Source: CAD feature listing. Evaluate the final solid. Frame: model axes, mm. A direction names the side the tool comes from. Give positions to 0.01 mm unless a question says otherwise; leave off trailing zeros. Write each loop counter-clockwise with the first axis right and the second up, starting at its lowest first coordinate (ties: lowest second). Pieces come first, ordered by that corner, then holes. Notation, with made-up numbers: (-13, 54) -> (21, 54) arc R28 cw to (21, 76) -> close; hole circle Ø9 at (-6.75, 55.5). An arc over 180 degrees is marked (long way). Use one line per item in the form item = value. Start each with the question number.
(1) Set-up query: faces 1 (the face through (-5, -2, 4)), 2 (the face through (-1.873, 3.367, 2.986)), 3 (the face through (-4.825, -7.192, 3.598)). Return all of +Z, -Z, +X, -X, +Y, -Y with unobstructed straight access to the full face (end or side cutting, diameter ignored); none if empty.
(2) Cut plane A-A, the plane z = 3.25. Count the separate pieces of the cut face and the enclosed holes in it, and give its area (3 significant figures).
(3) Material intervals for line 1 along Y through (x, z) = (-3, 1.75); line 2 along Z through (x, y) = (-3.5, 2.5); line 3 along Z through (x, y) = (-5.25, 8), sorted ascending. Write a range as from..to.
(4) Draft query along Z for faces 4 (the face through (-5, -2, 2)), 5 (the face through (-5.492, 5.648, 3.395)), 6 (the face through (-1.374, -10.002, 1.118)), 7 (the face through (-3.202, -7.94, 4.791)). Return one class per face: pulls with the +Z half, pulls with the -Z half, needs draft (parallel to the pull), parting line crosses it, or undercut.
(5) First-contact query: P1, Ø3, axis at x = -5.5, y = -9, coming from the -Z side; P2, Ø1.5, axis at y = -6, z = 5, coming from the +X side; P3, Ø1.6, axis at x = -3, y = 1, coming from the +Z side; P4, Ø4, axis at x = -3.5, y = -0.5, coming from the -Z side. Flat tips, straight axial feed; report the tip coordinate or a pass-through.
(6) Cut plane C-C, the plane x = -8.75. Output: boundary loops of the cut face in (y, z), and give its area (3 significant figures).
(7) Cut plane D-D, the plane y = -6. Output: boundary loops of the cut face in (x, z), and give its area (3 significant figures).
from build123d import *

# Parameters (mm, degrees)
BOSS_EXTRUDE2_DEPTH = 7
BOSS_EXTRUDE3_START = -2
BOSS_EXTRUDE3_DEPTH = 2
CUT_EXTRUDE1_REACH  = 20.032
SKETCH4_R           = 2.165
SKETCH6_R           = 3
CUT_EXTRUDE2_DEPTH  = 2.25


with BuildPart() as part:
    # Sketch2 → Boss-Extrude2 (new body)
    with BuildSketch(Plane.XY):
        with BuildLine():
            Line((-1.537034244, -5.640729849), (-1.207226003, -14.487186411))
            Line((-1.207226003, -14.487186411), (-7.804400539, -6.252306152))
            ThreePointArc((-7.804400539, -6.252306152), (-10, 0), (-7.804400539, 6.252306152))
            Line((-7.804400539, 6.252306152), (-2.239666493, 13.198449277))
            Line((-2.239666493, 13.198449277), (-1.909690796, 4.352324093))
            ThreePointArc((-1.909690796, 4.352324093), (-6.719838781, -0.830529263), (-1.537034244, -5.640729849))
        make_face()
    extrude(amount=BOSS_EXTRUDE2_DEPTH)

    # Sketch3 → Boss-Extrude3 (add)
    with BuildSketch(Plane.XY.offset(4).offset(BOSS_EXTRUDE3_START)):
        with BuildLine():
            Line((-1.909780577, 4.352320743), (-1.835249267, 2.353709953))
            ThreePointArc((-1.835249267, 2.353709953), (-4.721227993, -0.755997952), (-1.611655337, -3.642122406))
            Line((-1.611655337, -3.642122406), (-1.537124027, -5.640733196))
            ThreePointArc((-1.537124027, -5.640733196), (-6.719838781, -0.830529263), (-1.909780577, 4.352320743))
        make_face()
    extrude(amount=BOSS_EXTRUDE3_DEPTH)

    # Sketch4 → Cut-Extrude1 (cut, up to next)
    with BuildSketch(Plane(origin=(-1.744913711, -0.065088285, 0), x_dir=(0, 0, -1), z_dir=(0.9993050159682331, 0.03727579725142651, 0)), mode=Mode.PRIVATE) as cut_extrude1_sk1:
        with Locations(Location((-3.5, 8.846623232, 0), (0, 0, 90))):
            Circle(SKETCH4_R)
    cut_extrude1_tool1 = extrude(cut_extrude1_sk1.sketch, amount=-CUT_EXTRUDE1_REACH, mode=Mode.PRIVATE) & part.part
    # Sketch4 → Cut-Extrude1 (cut, up to next)
    with BuildSketch(Plane(origin=(-1.744913711, -0.065088285, 0), x_dir=(0, 0, -1), z_dir=(0.9993050159682331, 0.03727579725142651, 0)), mode=Mode.PRIVATE) as cut_extrude1_sk2:
        with Locations(Location((-3.5, -10.005816596, 0), (0, 0, 90))):
            Circle(SKETCH4_R)
    cut_extrude1_tool2 = extrude(cut_extrude1_sk2.sketch, amount=-CUT_EXTRUDE1_REACH, mode=Mode.PRIVATE) & part.part
    add(cut_extrude1_tool1.solids().sort_by_distance((-2.074679, 8.775387, 3.5))[0], mode=Mode.SUBTRACT)
    add(cut_extrude1_tool2.solids().sort_by_distance((-1.371939, -10.063951, 3.5))[0], mode=Mode.SUBTRACT)

    # Sketch6 → Cut-Extrude2 (cut, symmetric)
    with BuildSketch(Plane(origin=(-5.742133775, -0.214191474, 0), x_dir=(0, 0, 1), z_dir=(-0.9993050159682331, -0.03727579725142651, 0))):
        with Locations((3.5, -10.005816596)):
            Circle(SKETCH6_R)
        with Locations((3.5, 8.846623232)):
            Circle(SKETCH6_R)
    extrude(amount=CUT_EXTRUDE2_DEPTH, both=True, mode=Mode.SUBTRACT)


solid = part.part
Geometry says:
q1.face_1 = +Z, +X
q1.face_2 = +Z, -Z, +X, +Y
q1.face_3 = none
q2.separate_pieces = 3
q2.enclosed_holes = 0
q2.area = 89.4 mm^2
q3.line_1 = -12.25..-11.4, -8.85..-5.48, 4.19..7.47, 10.02..12.25
q3.line_2 = 2..4
q3.line_3 = 0..0.57, 6.43..7
q4.face_4 = pulls with the -Z half
q4.face_5 = undercut
q4.face_6 = needs draft
q4.face_7 = undercut
q5.P1 = 0
q5.P2 = -1.5
q5.P3 = through
q5.P4 = 2
q6.outline = (-4.84, 0) -> (4.84, 0) -> (4.84, 7) -> (-4.84, 7) -> close
q6.area = 67.8 mm^2
q7.outline = (-8, 0) -> (-1.52, 0) -> (-1.52, 7) -> (-8, 7) -> close
q7.area = 45.3 mm^2
